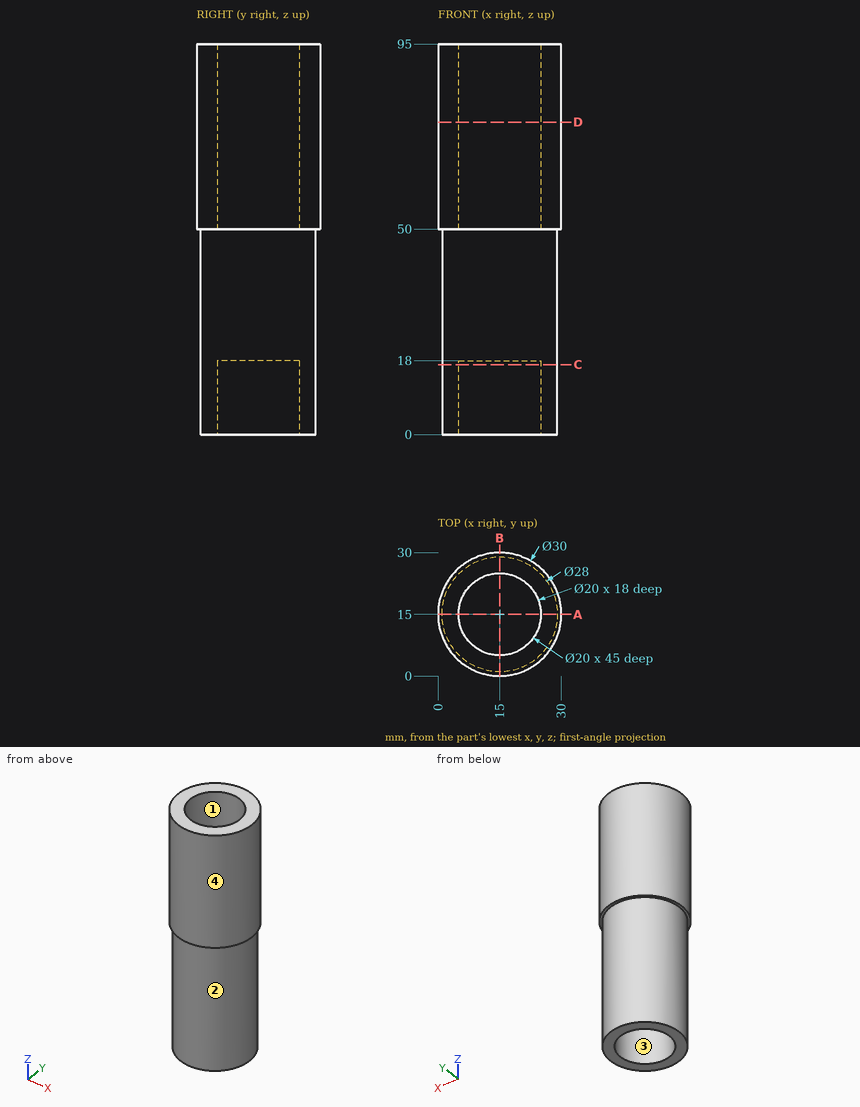
Answer from the drawing. Dimensions are ordinates in mm from the lowest x, y and z of the part. A direction names the side the tool comes from. Round coordinates to 2 decimals unless told otherwise and drop trailing zeros. Loops run counter-clockwise (first coordinate to the right, second up) from the corner with the lowest first, then second, coordinate; pieces in that order, holes last.
Q1. Section A-A on y = 15 is taken. Write down the section's boundary in (x, z).
Q2. Section D-D on z = 76 is taken. Write down the section's boundary in (x, y).
Q3. Which of the six approach directions +Z, -Z, +X, -X, +Y, -Y give full straight-line access (tool end or side, diameter ignored) to the marked faces 3 and 4?
Q4. Determine the mould class of the marked faces 1 and 2 for opening direction Y: released by +Y, released by -Y, zero draft, split by the parting line, or undercut.
Q5. Section C-C on z = 17 is taken. Write down the section's boundary in (x, y), and give its area (3 significant figures).
Q6. Each of these flat-tipped pins is pushed along its axis until it touches: pin 1 (1.5 mm diameter, centred on x = 26.5, z = 24, fed in from -Y); pin 2 (1.5 mm diameter, centred on x = 18, z = 24.5, fed in from -Y); pin 3 (6 mm diameter, centred on x = 19.5, y = 13, fed in from +Z). Where does it stop, or does it pass through?
Q7. Consider probe 1 along Y at (x, z) = (15, 86); probe 2 along Y at (x, z) = (15, 6.5); probe 3 along Z at (x, y) = (28.75, 9.5). Determine where each line is inside the solid, lowest interval first.
Output:
1. outline: (0, 50) - (1, 50) - (1, 0) - (5, 0) - (5, 18) - (25, 18) - (25, 0) - (29, 0) - (29, 50) - (30, 50) - (30, 95) - (25, 95) - (25, 50) - (5, 50) - (5, 95) - (0, 95) - close
2. outline: circle Ø30 at (15, 15); hole circle Ø20 at (15, 15)
3. face 3: -Z
3. face 4: +Z, -Z
4. face 1: undercut
4. face 2: split by the parting line
5. outline: circle Ø28 at (15, 15); hole circle Ø20 at (15, 15)
5. area: 302 mm2
6. pin 1: stops at y = 6.03
6. pin 2: stops at y = 1.18
6. pin 3: stops at z = 50
7. probe 1: y = 0 to 5, 25 to 30
7. probe 2: y = 1 to 5, 25 to 29
7. probe 3: z = 50 to 95
